from build123d import *

# Parameters (mm, degrees)
SKETCH1_W           = 70
SKETCH1_H           = 25
BOSS_EXTRUDE1_DEPTH = 5
CUT_EXTRUDE1_DEPTH  = 0.5
CUT_EXTRUDE2_DEPTH  = 75.498322129
CUT_EXTRUDE3_DEPTH  = 75.498322129
CUT_EXTRUDE4_DEPTH  = 75.498322129
CUT_EXTRUDE5_DEPTH  = 3
CUT_EXTRUDE6_DEPTH  = 3
CUT_EXTRUDE7_DEPTH  = 3
FILLET1_R           = 1


with BuildPart() as part:
    # Sketch1 → Boss-Extrude1 (new body)
    with BuildSketch(Plane.XY.offset(5)):
        with Locations((35, 12.5)):
            Rectangle(SKETCH1_W, SKETCH1_H)
    extrude(amount=-BOSS_EXTRUDE1_DEPTH)

    # Sketch2 → Cut-Extrude1 (cut)
    with BuildSketch(Plane.XY.offset(5)):
        with BuildLine():
            Line((38.9, 0), (38.9, 11))
            ThreePointArc((38.9, 11), (30, 19.9), (21.1, 11))
            Line((21.1, 11), (21.1, 0))
            Line((21.1, 0), (38.9, 0))
        make_face()
    extrude(amount=-CUT_EXTRUDE1_DEPTH, mode=Mode.SUBTRACT)

    # Sketch3 → Cut-Extrude2 (cut, through all)
    with BuildSketch(Plane(origin=(0, 0, 0), x_dir=(-1, 0, 0), z_dir=(0, 0, -1))):
        with BuildLine():
            Line((-36, 0), (-24, 0))
            Line((-24, 0), (-24, 11))
            ThreePointArc((-24, 11), (-30, 17), (-36, 11))
            Line((-36, 11), (-36, 0))
        make_face()
    extrude(amount=-CUT_EXTRUDE2_DEPTH, mode=Mode.SUBTRACT)

    # Sketch4 → Cut-Extrude3 (cut, through all)
    with BuildSketch(Plane(origin=(0, 0, 0), x_dir=(-1, 0, 0), z_dir=(0, 0, -1))):
        with BuildLine():
            Line((0, 8.5), (0, 13.5))
            Line((0, 13.5), (-9, 13.5))
            ThreePointArc((-9, 13.5), (-11.5, 11), (-9, 8.5))
            Line((-9, 8.5), (0, 8.5))
        make_face()
    extrude(amount=-CUT_EXTRUDE3_DEPTH, mode=Mode.SUBTRACT)

    # Sketch5 → Cut-Extrude4 (cut, through all)
    with BuildSketch(Plane(origin=(0, 0, 0), x_dir=(-1, 0, 0), z_dir=(0, 0, -1))):
        with BuildLine():
            Line((-52, 13.5), (-60, 13.5))
            ThreePointArc((-60, 13.5), (-62.5, 11), (-60, 8.5))
            Line((-60, 8.5), (-52, 8.5))
            ThreePointArc((-52, 8.5), (-49.5, 11), (-52, 13.5))
        make_face()
    extrude(amount=-CUT_EXTRUDE4_DEPTH, mode=Mode.SUBTRACT)

    # Sketch6 → Cut-Extrude5 (cut)
    with BuildSketch(Plane.XY.offset(5)):
        with BuildLine():
            Line((69, 5.5), (69, 19.5))
            ThreePointArc((69, 19.5), (66.6, 21.9), (64.2, 19.5))
            Line((64.2, 19.5), (64.2, 5.5))
            ThreePointArc((64.2, 5.5), (66.6, 3.1), (69, 5.5))
        make_face()
    extrude(amount=-CUT_EXTRUDE5_DEPTH, mode=Mode.SUBTRACT)

    # Sketch7 → Cut-Extrude6 (cut)
    with BuildSketch(Plane.XY.offset(5)):
        with BuildLine():
            Line((47.7, 5.5), (47.7, 19.5))
            ThreePointArc((47.7, 19.5), (44.3, 22.9), (40.9, 19.5))
            Line((40.9, 19.5), (40.9, 5.5))
            ThreePointArc((40.9, 5.5), (44.3, 2.1), (47.7, 5.5))
        make_face()
    extrude(amount=-CUT_EXTRUDE6_DEPTH, mode=Mode.SUBTRACT)

    # Sketch8 → Cut-Extrude7 (cut)
    with BuildSketch(Plane.XY.offset(5)):
        with BuildLine():
            Line((19.1, 5.5), (19.1, 19.5))
            ThreePointArc((19.1, 19.5), (16.2, 22.4), (13.3, 19.5))
            Line((13.3, 19.5), (13.3, 5.5))
            ThreePointArc((13.3, 5.5), (16.2, 2.6), (19.1, 5.5))
        make_face()
    extrude(amount=-CUT_EXTRUDE7_DEPTH, mode=Mode.SUBTRACT)

    # Fillet1
    fillet1_edges = [part.edges().sort_by_distance(p)[0] for p in [
        (36, 0, 2.25),
        (24, 0, 2.25),
        (0, 8.5, 2.5),
        (0, 13.5, 2.5),
        (70, 25, 2.5),
        (70, 0, 2.5),
        (0, 0, 2.5),
        (0, 25, 2.5),
    ]]
    fillet(fillet1_edges, radius=FILLET1_R)


solid = part.part
Design review of the part built by this model. Coordinates are the model's own, in mm. A direction names the side the tool comes from. Give positions to 0.01 mm unless a question says otherwise; leave off trailing zeros. Loops run counter-clockwise (first coordinate to the right, second up) from the corner with the lowest first, then second, coordinate; pieces in that order, holes last. Notation, with made-up numbers: (-31, -16.5) - (9, -16.5) arc R31 ccw to (9, 15.5) - close; hole circle Ø8 at (64.25, -32). An arc over 180 degrees is marked (long way). Write item = value, one per line.
1) Take a section at A-A on x = 16.2. State the section outline as (y, z) points.
Result sheet:
outline = (0, 0) - (25, 0) - (25, 5) - (22.4, 5) - (22.4, 2) - (2.6, 2) - (2.6, 5) - (0, 5) - close
2) Draft analysis for pull direction Y (two halves, no side actions). For faces 6 (the face through (12, 0, 3)), 7 (the face through (62.5, 11.1, 2.5)), 8 (the face through (36, 6, 2)), state which applies: +Y half, -Y half, draft (parallel to the pull), parting line (faces both ways), or undercut.
Result sheet:
face_6 = -Y half
face_7 = undercut
face_8 = draft
3) Tool access review of faces 1 (the face through (35, 25, 3)), 2 (the face through (69, 12, 4)), 3 (the face through (23.9, 12.3, 4.5)), 4 (the face through (56, 13.5, 2)), 5 (the face through (53, 0, 3)): name each direction out of +Z, -Z, +X, -X, +Y, -Y from which nothing blocks a thin tool from reaching the whole face with its end or side.
Result sheet:
face_1 = +Z, -Z, +X, -X, +Y
face_2 = +Z
face_3 = +Z, -Y
face_4 = +Z, -Z
face_5 = +Z, -Z, +X, -X, -Y
4) Take a section at B-B on z = 2.95. Count the separate pieces of the cut face and the enclosed holes in it, and give its area (3 significant figures).
Result sheet:
separate_pieces = 1
enclosed_holes = 4
area = 1,120 mm2
5) To check wall thickness, follow line 1 (X direction, y = 18.5, z = 3.1); line 2 (X direction, y = 7.5, z = 3.65); line 3 (X direction, y = 1.75, z = 2.8). State the ranges of each line that lie inside material, in increasing order.
Result sheet:
line_1 = 0 to 13.3, 19.1 to 40.9, 47.7 to 64.2, 69 to 70
line_2 = 0 to 13.3, 19.1 to 24, 36 to 40.9, 47.7 to 64.2, 69 to 70
line_3 = 0 to 24, 36 to 70
6) Clearance check with flat-ended pins moving along their axes: pin 1 Ø3.5 at (x, y) = (43, 17.5) entering from +Z; pin 2 Ø2.5 at (y, z) = (9.5, 3) entering from -X. State where each tip first meets the part, or that it passes through.
Result sheet:
pin_1 = 2
pin_2 = 0.34
7) Take a section at D-D on x = 30. State the section outline as (y, z) points.
Result sheet:
outline = (17, 0) - (25, 0) - (25, 5) - (19.9, 5) - (19.9, 4.5) - (17, 4.5) - close
8) Take a section at C-C on x = 66.6. State the section outline as (y, z) points.
Result sheet:
outline = (0, 0) - (25, 0) - (25, 5) - (21.9, 5) - (21.9, 2) - (3.1, 2) - (3.1, 5) - (0, 5) - close
